Read the model definition and answer for the solid it produces. Units are mm, in the model's axes. Round coordinates to 2 decimals unless told otherwise and drop trailing zeros. Write each loop counter-clockwise with the first axis right and the second up, starting at its lowest first coordinate (ties: lowest second). Pieces come first, ordered by that corner, then holes.
from build123d import *

# Parameters (mm, degrees)
SZKIC1_R                    = 1.5
DODANIE_WYCI_GNI_CIE1_DEPTH = 60
SZKIC2_R                    = 2
DODANIE_WYCI_GNI_CIE2_DEPTH = 1
ZAOKR_GLENIE1_R             = 1
DODANIE_WYCI_GNI_CIE3_START = 1
SZKIC3_R                    = 2
DODANIE_WYCI_GNI_CIE3_DEPTH = 1
ZAOKR_GLENIE2_R             = 1


with BuildPart() as part:
    # Szkic1 → Dodanie-wyciągnięcie1 (new body)
    with BuildSketch(Plane(origin=(0, 0, 0), x_dir=(1, 0, 0), z_dir=(0, 1, 0))):
        with Locations(Location((0, 0, 0), (0, 0, 270))):
            Circle(SZKIC1_R)
    extrude(amount=DODANIE_WYCI_GNI_CIE1_DEPTH)

    # Szkic2 → Dodanie-wyciągnięcie2 (add)
    with BuildSketch(Plane(origin=(0, 60, 0), x_dir=(1, 0, 0), z_dir=(0, 1, 0))):
        with Locations(Location((0, 0, 0), (0, 0, 270))):
            Circle(SZKIC2_R)
    extrude(amount=DODANIE_WYCI_GNI_CIE2_DEPTH)

    # Zaokrąglenie1
    zaokr_glenie1_edges = [part.edges().sort_by_distance(p)[0] for p in [
        (0, 61, -2),
    ]]
    fillet(zaokr_glenie1_edges, radius=ZAOKR_GLENIE1_R - 0.0001)  # a hair under: the kernel refuses the full size

    # Szkic3 → Dodanie-wyciągnięcie3 (add)
    with BuildSketch(Plane.XZ.offset(DODANIE_WYCI_GNI_CIE3_START)):
        with Locations(Location((0, 0, 0), (0, 0, 270))):
            Circle(SZKIC3_R)
    extrude(amount=-DODANIE_WYCI_GNI_CIE3_DEPTH)

    # Zaokrąglenie2
    zaokr_glenie2_edges = [part.edges().sort_by_distance(p)[0] for p in [
        (0, -1, 2),
    ]]
    fillet(zaokr_glenie2_edges, radius=ZAOKR_GLENIE2_R - 0.0001)  # a hair under: the kernel refuses the full size


solid = part.part
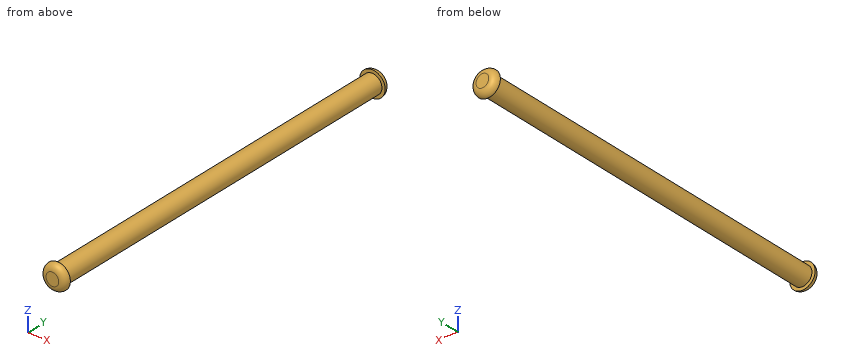
Q1. Straight lines are drawn through the part: probe 1 along X at (y, z) = (28, 0.05); probe 2 along Y at (x, z) = (-1.15, 1.55); probe 3 along Y at (x, z) = (1.65, -0.1). For each, find the intervals that lie inside material, in ascending order.
Verdict:
probe 1: x = -1.5 to 1.5
probe 2: y = -0.37 to 0, 60 to 60.37
probe 3: y = -0.76 to 0, 60 to 60.76
Q2. Flat-ended cylindrical pins translate along their axes: pin 1 Ø1 at (y, z) = (51.5, 1.5) entering from -X; pin 2 Ø1 at (x, y) = (1.5, 26) entering from +Z; pin 3 Ø1 at (x, y) = (0.5, 9) entering from +Z. Find the tip coordinate at first contact, or state that the pin passes through.
Verdict:
pin 1: stops at x = -1.12
pin 2: stops at z = 1.12
pin 3: stops at z = 1.5
Q3. Section C-C (y = 24.5) is taken. Determine the outline of the cut face in (x, z).
Verdict:
outline: circle Ø3 at (0, 0)
